from build123d import *

# Parameters (mm, degrees)
EXTRUDE_THIN1_DEPTH = 152.4
CUT_EXTRUDE1_DEPTH  = 3
CUT_EXTRUDE2_DEPTH  = 3
LPATTERN1_COUNT     = 4
LPATTERN1_PITCH     = 45
LPATTERN2_COUNT     = 4
LPATTERN2_PITCH     = 45


with BuildPart() as part:
    # Sketch1 → Extrude-Thin1 (new body)
    with BuildSketch(Plane.XY):
        Polygon((0, 20), (0, 0), (20, 0), (20, 3), (3, 3), (3, 20), align=None)
    extrude(amount=EXTRUDE_THIN1_DEPTH)

    # Sketch2 → Cut-Extrude1 (cut)
    with BuildSketch(Plane(origin=(0, 3, 0), x_dir=(1, 0, 0), z_dir=(0, 1, 0))):
        with BuildLine():
            Line((7.25, -147.6), (7.25, -142.6))
            ThreePointArc((7.25, -142.6), (10, -139.85), (12.75, -142.6))
            Line((12.75, -142.6), (12.75, -147.6))
            ThreePointArc((12.75, -147.6), (10, -150.35), (7.25, -147.6))
        make_face()
        with BuildLine():
            Line((12.75, -120.1), (12.75, -125.1))
            ThreePointArc((12.75, -125.1), (10, -127.85), (7.25, -125.1))
            Line((7.25, -125.1), (7.25, -120.1))
            ThreePointArc((7.25, -120.1), (10, -117.35), (12.75, -120.1))
        make_face()
        with BuildLine():
            Line((7.25, -102.6), (7.25, -97.6))
            ThreePointArc((7.25, -97.6), (10, -94.85), (12.75, -97.6))
            Line((12.75, -97.6), (12.75, -102.6))
            ThreePointArc((12.75, -102.6), (10, -105.35), (7.25, -102.6))
        make_face()
    cut_extrude1 = extrude(amount=-CUT_EXTRUDE1_DEPTH, mode=Mode.SUBTRACT)

    # Sketch3 → Cut-Extrude2 (cut)
    with BuildSketch(Plane(origin=(3, 0, 0), x_dir=(0, 0, -1), z_dir=(1, 0, 0))):
        with BuildLine():
            Line((-147.6, 17.75), (-142.6, 17.75))
            ThreePointArc((-142.6, 17.75), (-139.85, 15), (-142.6, 12.25))
            Line((-142.6, 12.25), (-147.6, 12.25))
            ThreePointArc((-147.6, 12.25), (-150.35, 15), (-147.6, 17.75))
        make_face()
        with BuildLine():
            Line((-125.1, 17.75), (-120.1, 17.75))
            ThreePointArc((-120.1, 17.75), (-117.35, 15), (-120.1, 12.25))
            Line((-120.1, 12.25), (-125.1, 12.25))
            ThreePointArc((-125.1, 12.25), (-127.85, 15), (-125.1, 17.75))
        make_face()
        with BuildLine():
            Line((-102.6, 17.75), (-97.6, 17.75))
            ThreePointArc((-97.6, 17.75), (-94.85, 15), (-97.6, 12.25))
            Line((-97.6, 12.25), (-102.6, 12.25))
            ThreePointArc((-102.6, 12.25), (-105.35, 15), (-102.6, 17.75))
        make_face()
    cut_extrude2 = extrude(amount=-CUT_EXTRUDE2_DEPTH, mode=Mode.SUBTRACT)

    # LPattern1: Cut-Extrude1 ×4
    with Locations(*[(0, 0, -i * LPATTERN1_PITCH) for i in range(1, LPATTERN1_COUNT)]):
        add(cut_extrude1, mode=Mode.SUBTRACT)

    # LPattern2: Cut-Extrude2 ×4
    with Locations(*[(0, 0, -i * LPATTERN2_PITCH) for i in range(1, LPATTERN2_COUNT)]):
        add(cut_extrude2, mode=Mode.SUBTRACT)


solid = part.part
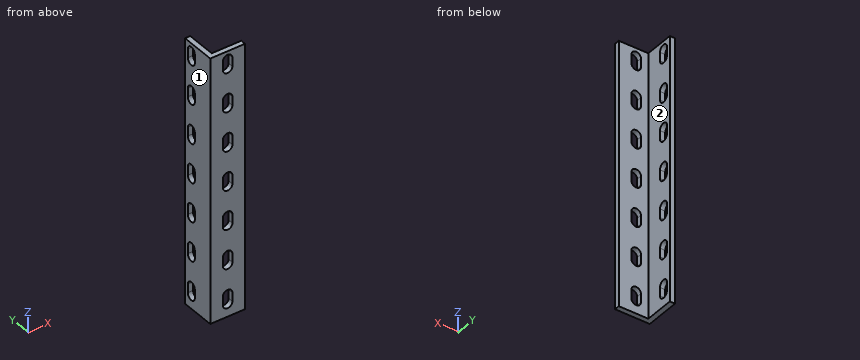
Can you work these out from the model? Positions are in its coordinate system, mm. Face numbers are marked on the shaded views. A direction names the side the tool comes from. Give positions to 0.01 mm unless a question says otherwise; leave off trailing zeros. Loops run counter-clockwise (first coordinate to the right, second up) from the corner with the lowest first, then second, coordinate; pieces in that order, holes last. Notation, with made-up numbers: (42, -32.5) -> (51, -32.5) arc R18 ccw to (51, -0.5) -> close; hole circle Ø7 at (50.5, -8.5). An arc over 180 degrees is marked (long way). Return JSON: item names as keys, results as strings.
Q1. For pin 1 Ø2 at (y, z) = (10.5, 20) entering from +X; pin 2 Ø10 at (x, y) = (13, 11.5) entering from -Z, each with a flat end and sliding along its axis, tell me the tip position at first contact or that it passes through.
Checks:
{"pin 1": "stops at x = 3", "pin 2": "passes through"}
Q2. I want a section at A-A, the plane y = 15. Count the separate pieces of the cut face and the enclosed holes in it, then the cut area to 3 significant figures.
Checks:
{"separate pieces": "8", "enclosed holes": "0", "area": "237 mm2"}
Q3. I want a section at D-D, the plane z = 67. List the corners of the cut face in (x, y) for me, then the cut area to 3 significant figures.
Checks:
{"outline": "(0, 0) -> (20, 0) -> (20, 3) -> (3, 3) -> (3, 20) -> (0, 20) -> close", "area": "111 mm2"}
Q4. I need wall thicknesses on probe 1 along X at (y, z) = (5, 91.5); probe 2 along X at (y, z) = (2.25, 127). Which ranges of each line are inside material? Lowest first, please.
Checks:
{"probe 1": "x = 0 to 3", "probe 2": "x = 0 to 8.01, 11.99 to 20"}
Q5. On a 3-axis mill with a long thin cutter (end or side, diameter ignored), from which of +Z, -Z, +X, -X, +Y, -Y can I reach the whole of each face in a straight line? I mean the marked faces 1 and 2. Say none if no direction works.
Checks:
{"face 1": "+Z, -Z, -X, +Y, -Y", "face 2": "+Z, -Z, +X, +Y"}
